```python
from build123d import *

# Parameters (mm, degrees)
SKETCH1_W           = 45
SKETCH1_H           = 65
BOSS_EXTRUDE1_DEPTH = 5
BOSS_EXTRUDE2_DEPTH = 20
BOSS_EXTRUDE3_DEPTH = 5.3


with BuildPart() as part:
    # Sketch1 → Boss-Extrude1 (new body)
    with BuildSketch(Plane.XY):
        with Locations((2.886207951, -16.286739239)):
            Rectangle(SKETCH1_W, SKETCH1_H)
    extrude(amount=BOSS_EXTRUDE1_DEPTH)

    # Sketch4 → Boss-Extrude2 (add)
    with BuildSketch(Plane(origin=(0, 0, 0), x_dir=(-1, 0, 0), z_dir=(0, 0, -1))):
        with BuildLine():
            Line((16.363792049, -6.036739239), (16.363792049, -26.536739239))
            ThreePointArc((16.363792049, -26.536739239), (-2.886207951, -45.786739239), (-22.136207951, -26.536739239))
            Line((-22.136207951, -26.536739239), (-22.136207951, -6.036739239))
            ThreePointArc((-22.136207951, -6.036739239), (-2.886207951, 13.213260761), (16.363792049, -6.036739239))
        make_face()
        with BuildLine():
            Line((7.863792049, -6.036739239), (7.863792049, -26.536739239))
            ThreePointArc((7.863792049, -26.536739239), (-2.886207951, -37.286739239), (-13.636207951, -26.536739239))
            Line((-13.636207951, -26.536739239), (-13.636207951, -6.036739239))
            ThreePointArc((-13.636207951, -6.036739239), (-2.886207951, 4.713260761), (7.863792049, -6.036739239))
        make_face(mode=Mode.SUBTRACT)
    extrude(amount=BOSS_EXTRUDE2_DEPTH)


with BuildPart() as body_2:
    # Sketch6 → Boss-Extrude3 (new body)
    with BuildSketch(Plane(origin=(0, 0, 0), x_dir=(-1, 0, 0), z_dir=(0, 0, -1))):
        with BuildLine():
            Line((16.363792049, -6.036739239), (16.363792049, -26.536739239))
            ThreePointArc((16.363792049, -26.536739239), (-2.886207951, -45.786739239), (-22.136207951, -26.536739239))
            Line((-22.136207951, -26.536739239), (-22.136207951, -6.036739239))
            ThreePointArc((-22.136207951, -6.036739239), (-2.886207951, 13.213260761), (16.363792049, -6.036739239))
        make_face()
        with BuildLine():
            Line((12.029792049, -6.036739239), (12.029792049, -26.536739239))
            ThreePointArc((12.029792049, -26.536739239), (-2.886207951, -41.452739239), (-17.802207951, -26.536739239))
            Line((-17.802207951, -26.536739239), (-17.802207951, -6.036739239))
            ThreePointArc((-17.802207951, -6.036739239), (-2.886207951, 8.879260761), (12.029792049, -6.036739239))
        make_face(mode=Mode.SUBTRACT)
    extrude(amount=BOSS_EXTRUDE3_DEPTH)


with BuildPart() as body_2_1:
    # Body-Move/Copy1: read off the stored shape, not the designer's step
    # Body-Move/Copy1: moved
    add(body_2.part.moved(Location((0, 0, -8))))


with BuildPart() as part_1:
    add(part.part)

    # Combine1: cut body 2
    add(body_2_1.part, mode=Mode.SUBTRACT)


solid = part_1.part
```
Build history of the part. All positions in model axes, mm. A direction names the side the tool comes from. Give positions to 0.01 mm unless a question says otherwise; leave off trailing zeros. Loops run counter-clockwise (first coordinate to the right, second up) from the corner with the lowest first, then second, coordinate; pieces in that order, holes last.
1) Two-plate mould, pull along X, no slides. Class faces 4 (the face through (18, -16, -13.3)), 5 (the face through (22.136, -16, -17)), 6 (the face through (3.12, 4.71, -9.86)), 7 (the face through (2.463, -45.782, -3.944)): released by +X, released by -X, zero draft, split by the parting line, or undercut.
Values follow:
face 4: zero draft
face 5: released by +X
face 6: undercut
face 7: split by the parting line
2) Band-saw the part on D-D on x = 10.5. List the corners of the cut face in (y, z).
Values follow:
outline: (-48.79, 0) - (-44.22, 0) - (-44.22, -8) - (-39.36, -8) - (-39.36, -13.3) - (-44.22, -13.3) - (-44.22, -20) - (-34.13, -20) - (-34.13, 0) - (1.55, 0) - (1.55, -20) - (11.64, -20) - (11.64, -13.3) - (6.79, -13.3) - (6.79, -8) - (11.64, -8) - (11.64, 0) - (16.21, 0) - (16.21, 5) - (-48.79, 5) - close
3) 3-axis set-ups, long thin cutter, end or side, ignore diameter. For faces 1 (the face through (3, -16, 0)), 2 (the face through (2.463, -45.782, -16.603)), 3 (the face through (-16.364, -16, -17)): which of +Z, -Z, +X, -X, +Y, -Y reach the whole face in a straight line?
Values follow:
face 1: -Z
face 2: -Z, -Y
face 3: -Z, -X, +Y, -Y
4) Band-saw the part on A-A on y = -17.5. List the corners of the cut face in (x, z).
Values follow:
outline: (-19.61, 0) - (-16.36, 0) - (-16.36, -8) - (-12.03, -8) - (-12.03, -13.3) - (-16.36, -13.3) - (-16.36, -20) - (-7.86, -20) - (-7.86, 0) - (13.64, 0) - (13.64, -20) - (22.14, -20) - (22.14, -13.3) - (17.8, -13.3) - (17.8, -8) - (22.14, -8) - (22.14, 0) - (25.39, 0) - (25.39, 5) - (-19.61, 5) - close
5) Band-saw the part on B-B on z = -18.25. List the corners of the cut face in (x, y), then the cut area to 3 significant figures.
Values follow:
outline: (-16.36, -26.54) arc R19.25 ccw to (22.14, -26.54) - (22.14, -6.04) arc R19.25 ccw to (-16.36, -6.04) - close; hole (-7.86, -26.54) arc R10.75 ccw to (13.64, -26.54) - (13.64, -6.04) arc R10.75 ccw to (-7.86, -6.04) - close
area: 1,150 mm2
6) Probe line 1 along X through (y, z) = (-16, -10.5); line 2 along X through (y, z) = (-11, -17.5); line 3 along Z through (x, y) = (19.5, -4). List the from-to ranges inside material, lowest first.
Values follow:
line 1: x = -12.03 to -7.86, 13.64 to 17.8
line 2: x = -16.36 to -7.86, 13.64 to 22.14
line 3: z = -20 to -13.3, -8 to 5
7) Band-saw the part on C-C on x = -13. List the corners of the cut face in (y, z), then the cut area to 3 significant figures.
Values follow:
outline: (-48.79, 0) - (-37.41, 0) - (-37.41, -8) - (4.83, -8) - (4.83, 0) - (16.21, 0) - (16.21, 5) - (-48.79, 5) - close; (-37.41, -20) - (4.83, -20) - (4.83, -13.3) - (-37.41, -13.3) - close
area: 946 mm2
8) Drop flat-ended pins along their axis: P1, Ø2, axis at y = -16.5, z = -18, coming from the +X side; P2, Ø10, axis at x = 19.5, z = -13, coming from the +Y side; P3, Ø1.5, axis at x = -12.5, z = -8.5, coming from the -Y side. Give the stop position or say it passes through.
Values follow:
P1: stops at x = 22.14
P2: stops at y = 9.31
P3: stops at y = -38.81
